Design review of the part built by this model. Coordinates are the model's own, in mm. Face numbers are marked on the shaded views. A direction names the side the tool comes from. Coordinates: 2 decimals unless noted, no trailing zeros. Loops run counter-clockwise (first coordinate to the right, second up) from the corner with the lowest first, then second, coordinate; pieces in that order, holes last. Notation, with made-up numbers: (-19.5, 65) -> (17.5, 65) arc R10 cw to (17.5, 73) -> close; hole circle Ø1 at (88, 56.5). An arc over 180 degrees is marked (long way). One line per item, written item: value. Start each with the question number.
1. Machinability: for the marked faces 4, 5, 6, 7 and 8, which of the approach directions +Z, -Z, +X, -X, +Y, -Y give a long, thin tool a straight path to every point of the face, cutting with its end or side? Answer none if there is none.
2. Add section C-C on y = -2. Write out the cut boundary in (x, z), plus the area to 3 significant figures.
3. Insertion check: pin 1 (6 mm diameter, centred on x = 0.5, y = -5.5, fed in from +Z); pin 2 (2 mm diameter, centred on y = 8.5, z = -6.5, fed in from -X) (3 decimals); pin 3 (10 mm diameter, centred on x = -4.5, z = -10, fed in from -Y); pin 4 (4 mm diameter, centred on x = -2, y = -6, fed in from -Z). Each pin has a flat end and moves straight along its axis. Give the tip position at first contact, or say it passes through.
4. For probe 1 along Z at (x, y) = (4, -3.75); probe 2 along Y at (x, z) = (-1, -7); probe 3 along Y at (x, z) = (0.5, -5.5), list the stretches that pass through material, from the lowest coordinate up.
5. Add section D-D on y = 5.5. Write out the cut boundary in (x, z), plus the area to 3 significant figures.
6. Draft analysis for pull direction Y (two halves, no side actions). For the marked faces 1, 2 and 3, state which applies: pulls with the +Y half, pulls with the -Y half, needs draft (parallel to the pull), parting line crosses it, or undercut.
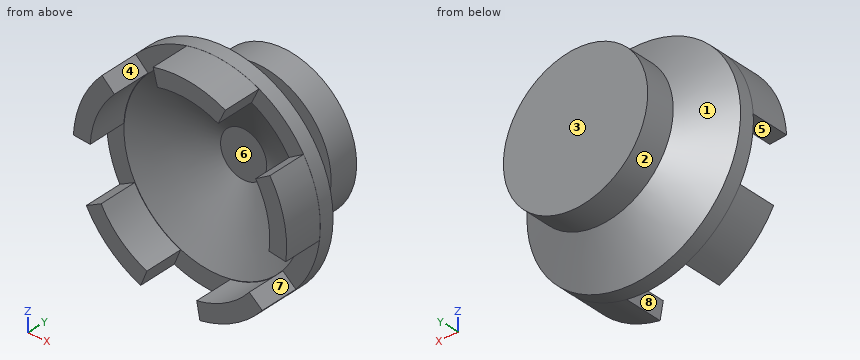
```python
from build123d import *

# Parameters (mm, degrees)
EXTRUDE_START   = 3.5
EXTRUDE_3_DEPTH = 9
SKETCH_4_R      = 12.5
EXTRUDE_4_DEPTH = 5


with BuildPart() as part:
    # 草圖1 → 旋轉1 (revolve)
    with BuildSketch(Plane.XY):
        Polygon((0, 6.154761905), (0, 3.154761905), (4, 3.154761905), (15.5, -2.757936508), (18.5, -2.757936508), (18.5, -0.257936508), (4.354320213, 6.154761905), align=None)
    revolve(axis=Axis((0, 6.154761905, 0), (0, -1, 0)))

    # 草圖2 → 填料-伸長3 (add)
    with BuildSketch(Plane.XZ.offset(-3.154761905).offset(EXTRUDE_START)):
        with BuildLine():
            Line((-4.628340567, 17.895656272), (-3.896757076, 15.066960653))
            ThreePointArc((-3.896757076, 15.066960653), (1.45159982, 15.49486615), (6.627417355, 14.081028309))
            Line((6.627417355, 14.081028309), (7.871659433, 16.724623391))
            ThreePointArc((7.871659433, 16.724623391), (1.724125523, 18.40389744), (-4.628340567, 17.895656272))
        make_face()
        with BuildLine():
            Line((18.338538597, -2.318200146), (15.439838321, -1.951771416))
            ThreePointArc((15.439838321, -1.951771416), (15.185062434, 3.407623498), (13.12536695, 8.361983105))
            Line((13.12536695, 8.361983105), (15.58954462, 9.931875369))
            ThreePointArc((15.58954462, 9.931875369), (18.035930673, 4.047376258), (18.338538597, -2.318200146))
        make_face()
        with BuildLine():
            Line((3.462180724, -18.157349874), (2.914927508, -15.287289382))
            ThreePointArc((2.914927508, -15.287289382), (7.933284886, -13.388839007), (12.008679966, -9.898970881))
            Line((12.008679966, -9.898970881), (14.263209011, -11.757419722))
            ThreePointArc((14.263209011, -11.757419722), (9.422692651, -15.902481347), (3.462180724, -18.157349874))
        make_face()
        with BuildLine():
            Line((-16.198793235, -8.903659222), (-13.638314046, -7.496293018))
            ThreePointArc((-13.638314046, -7.496293018), (-10.282022732, -11.682381074), (-5.703594571, -14.479883563))
            Line((-5.703594571, -14.479883563), (-6.774396662, -17.198360377))
            ThreePointArc((-6.774396662, -17.198360377), (-12.212386349, -13.875650236), (-16.198793235, -8.903659222))
        make_face()
        with BuildLine():
            Line((-13.47358552, 12.65458585), (-11.343869138, 10.654325507))
            ThreePointArc((-11.343869138, 10.654325507), (-14.287924407, 6.168730433), (-15.533695269, 0.949910686))
            Line((-15.533695269, 0.949910686), (-18.450016402, 1.128248458))
            ThreePointArc((-18.450016402, 1.128248458), (-16.970362498, 7.326857885), (-13.47358552, 12.65458585))
        make_face()
    extrude(amount=EXTRUDE_3_DEPTH)

    # 草圖4 → 填料-伸長4 (add)
    with BuildSketch(Plane(origin=(0, 6.154761905, 0), x_dir=(1, 0, 0), z_dir=(0, 1, 0))):
        with Locations(Location((0, 0, 0), (0, 0, 180))):
            Circle(SKETCH_4_R)
    extrude(amount=EXTRUDE_4_DEPTH)


solid = part.part
```
Worked answers:
1. face 4: +Z, +X, -Y
1. face 5: -X, -Y
1. face 6: -Y
1. face 7: +X, -Y
1. face 8: -Z, -Y
2. outline: circle Ø37 at (0, 0); hole circle Ø28.05 at (0, 0)
2. area: 457 mm²
3. pin 1: stops at z = 18.5
3. pin 2: stops at x = -11.225
3. pin 3: stops at y = -9.35
3. pin 4: stops at z = 15.07
4. probe 1: z = -18.05 to -15.04, 15.04 to 18.05
4. probe 2: y = 1.58 to 4.92, 6.15 to 11.15
4. probe 3: y = 2.37 to 5.63, 6.15 to 11.15
5. outline: circle Ø11.6 at (0, 0)
5. area: 106 mm²
6. face 1: undercut
6. face 2: needs draft
6. face 3: pulls with the +Y half
